from build123d import *

# Parameters (mm, degrees)
SKETCH1_W                     = 199.5
SKETCH1_H                     = 249.5
SKETCH1_W_2                   = 189.5
SKETCH1_H_2                   = 239.5
SKETCH1_W_3                   = 179.5
SKETCH1_H_3                   = 229.5
BOSS_EXTRUDE1_DEPTH           = 5
SKETCH1_3_W                   = 189.5
SKETCH1_3_H                   = 239.5
SKETCH1_3_W_2                 = 179.5
SKETCH1_3_H_2                 = 229.5
BOSS_EXTRUDE2_DEPTH           = 15
M3_CLEARANCE_HOLE1_AT_2_COUNT = 2
M3_CLEARANCE_HOLE1_AT_2_PITCH = 160


with BuildPart() as part:
    # Sketch1 → Boss-Extrude1 (new body)
    with BuildSketch(Plane(origin=(0, 0, 0), x_dir=(1, 0, 0), z_dir=(0, 1, 0))):
        Rectangle(SKETCH1_W, SKETCH1_H)
        Rectangle(SKETCH1_W_2, SKETCH1_H_2, mode=Mode.SUBTRACT)
        Rectangle(SKETCH1_W_2, SKETCH1_H_2)
        Rectangle(SKETCH1_W_3, SKETCH1_H_3, mode=Mode.SUBTRACT)
        Rectangle(SKETCH1_W_3, SKETCH1_H_3)
    extrude(amount=BOSS_EXTRUDE1_DEPTH)

    # Sketch1_3 → Boss-Extrude2 (add)
    with BuildSketch(Plane(origin=(0, 0, 0), x_dir=(1, 0, 0), z_dir=(0, 1, 0))):
        Rectangle(SKETCH1_3_W, SKETCH1_3_H)
        Rectangle(SKETCH1_3_W_2, SKETCH1_3_H_2, mode=Mode.SUBTRACT)
    extrude(amount=-BOSS_EXTRUDE2_DEPTH)

    # Sketch4 → M3 Clearance Hole1 (revolve, cut)
    with BuildSketch(Plane(origin=(-80, -8, 0), x_dir=(0, 1, 0), z_dir=(1, 0, 0))):
        Polygon((0, 0), (0, 124.75), (1.7, 124.75), (1.7, 0.025), (1.725, 0), align=None)
    m3_clearance_hole1 = revolve(axis=Axis((-80, -8, -6.35), (0, 0, 1)), mode=Mode.SUBTRACT)

    # M3 Clearance Hole1 at 2: M3 Clearance Hole1 ×2
    with Locations(*[(i * M3_CLEARANCE_HOLE1_AT_2_PITCH, 0, 0) for i in range(1, M3_CLEARANCE_HOLE1_AT_2_COUNT)]):
        add(m3_clearance_hole1, mode=Mode.SUBTRACT)

    # Mirror1: M3 Clearance Hole1 across plane
    add(m3_clearance_hole1.mirror(Plane.XY), mode=Mode.SUBTRACT)

    # Mirror1 copy 1 sketch → Mirror1 copy 1 (revolve, cut)
    with BuildSketch(Plane(origin=(80, -8, 0), x_dir=(0, 1, 0), z_dir=(1, 0, 0))):
        Polygon((0, 0), (0, -124.75), (1.7, -124.75), (1.7, -0.025), (1.725, 0), align=None)
    revolve(axis=Axis((80, -8, 6.35), (0, 0, 1)), mode=Mode.SUBTRACT)


solid = part.part
Work out the finished part from the listing and answer in its coordinate system (mm). A direction names the side the tool comes from. Round coordinates to 2 decimals unless told otherwise and drop trailing zeros. Loops run counter-clockwise (first coordinate to the right, second up) from the corner with the lowest first, then second, coordinate; pieces in that order, holes last. Notation, with made-up numbers: M -34.75,-38.75 L 6.25,-38.75 A12 ccw 6.25,-15.75 Z; hole C -12.75,49.25 d3. An arc over 180 degrees is marked long. One line per question, with ' | ' between items. Start each with the question number.
(1) For a pull along X with two mould halves and no side action, classify faces 1 (the face through (-99.75, 2, 2)), 2 (the face through (-1, -7, 114.75)), 3 (the face through (-1, -7, 119.75)), 4 (the face through (-1, -7, -114.75)) as released by +X, released by -X, zero draft, split by the parting line, or undercut.
(2) Flat-ended cylindrical pins translate along their axes: pin 1 Ø6 at (x, y) = (69.5, -11.5) entering from +Z; pin 2 Ø2 at (x, z) = (-39.5, -97) entering from -Y; pin 3 Ø2 at (x, y) = (66.5, -7.5) entering from -Z; pin 4 Ø2.5 at (x, y) = (80, -8) entering from +Z. Find the tip coordinate at first contact, or state that the pin passes through.
(3) A cutting plane is placed at A-A on z = -50.5. Write down the section's boundary in (x, y), plus the area to 3 significant figures.
(4) A tool of negligible diameter and unlimited length cuts with its end or side. For faces 5 (the face through (-94.75, -7, 2)), 6 (the face through (-1, 0, -2)), 7 (the face through (-1, -7, -119.75)), 8 (the face through (94.75, -7, 2)), from which of +Z, -Z, +X, -X, +Y, -Y can it reach the whole face along a straight path? Write none if from no direction.
(5) A cutting plane is placed at B-B on x = 55.5. Write down the section's boundary in (y, z), plus the area to 3 significant figures.
(6) Find the intervals of material crossed by line 1 (X direction, y = -8, z = -118); line 2 (Z direction, x = -12.5, y = -10.5); line 3 (Y direction, x = 80, z = -117), in increasing order.
Geometry check:
1) face 1: released by -X | face 2: undercut | face 3: zero draft | face 4: undercut
2) pin 1: stops at z = 119.75 | pin 2: stops at y = 0 | pin 3: stops at z = -119.75 | pin 4: passes through
3) outline: M -99.75,0 L -94.75,0 L -94.75,-15 L -89.75,-15 L -89.75,0 L 89.75,0 L 89.75,-15 L 94.75,-15 L 94.75,0 L 99.75,0 L 99.75,5 L -99.75,5 Z | area: 1,150 mm²
4) face 5: +Z, -Z, -X, -Y | face 6: -Y | face 7: -Z, +X, -X, -Y | face 8: +Z, -Z, +X, -Y
5) outline: M -15,-119.75 L 0,-119.75 L 0,-124.75 L 5,-124.75 L 5,124.75 L 0,124.75 L 0,119.75 L -15,119.75 L -15,114.75 L 0,114.75 L 0,-114.75 L -15,-114.75 Z | area: 1,400 mm²
6) line 1: x = -94.75 to -81.7, -78.3 to 78.3, 81.7 to 94.75 | line 2: z = -119.75 to -114.75, 114.75 to 119.75 | line 3: y = -15 to -9.7, -6.3 to 5
